CAD build for the part. Positions are in the model's coordinates, mm. A direction names the side the tool comes from. Give positions to 0.01 mm unless a question says otherwise; leave off trailing zeros. Loops run counter-clockwise (first coordinate to the right, second up) from the corner with the lowest first, then second, coordinate; pieces in that order, holes last. Notation, with made-up numbers: (-38, 18) - (21, 18) arc R23 cw to (21, 41) - close; hole circle Ø8 at (60, -14). An arc over 180 degrees is marked (long way). Return JSON: item names as keys, results as strings.
from build123d import *

# Parameters (mm, degrees)
BOX069_W          = 2
BOX069_H          = 2
BOX069_DEPTH      = 2
BOX070_W          = 2
BOX070_H          = 2
BOX070_DEPTH      = 2
CYLINDER040_R     = 0.75
CYLINDER040_DEPTH = 10
CYLINDER037_R     = 0.75
CYLINDER037_DEPTH = 10
BOX038_W          = 5
BOX038_H          = 11
BOX038_DEPTH      = 3.2
BOX003_W          = 4
BOX003_H          = 19
BOX003_DEPTH      = 5
FILLET_R          = 1
FILLET001_R       = 1
FILLET002_R       = 1
FILLET003_R       = 1


with BuildPart() as cubo069:
    # Box069 → Box069 (new body)
    with BuildSketch(Plane(origin=(-27, 67, 43), x_dir=(1, 0, 0), z_dir=(0, 0, 1))):
        with Locations((1, 1)):
            Rectangle(BOX069_W, BOX069_H)
    extrude(amount=BOX069_DEPTH)


with BuildPart() as cubo070:
    # Box070 → Box070 (new body)
    with BuildSketch(Plane(origin=(-27, 50, 43), x_dir=(1, 0, 0), z_dir=(0, 0, 1))):
        with Locations((1, 1)):
            Rectangle(BOX070_W, BOX070_H)
    extrude(amount=BOX070_DEPTH)


with BuildPart() as cilindro040:
    # Cylinder040 → Cylinder040 (new body)
    with BuildSketch(Plane(origin=(-26, 66, 42), x_dir=(1, 0, 0), z_dir=(0, 0, 1))):
        Circle(CYLINDER040_R)
    extrude(amount=CYLINDER040_DEPTH)


with BuildPart() as cilindro037:
    # Cylinder037 → Cylinder037 (new body)
    with BuildSketch(Plane(origin=(-26, 53, 42), x_dir=(1, 0, 0), z_dir=(0, 0, 1))):
        Circle(CYLINDER037_R)
    extrude(amount=CYLINDER037_DEPTH)


with BuildPart() as cubo038:
    # Box038 → Box038 (new body)
    with BuildSketch(Plane(origin=(-28.5, 54, 51), x_dir=(1, 0, 0), z_dir=(0, 0, 1))):
        with Locations((2.5, 5.5)):
            Rectangle(BOX038_W, BOX038_H)
    extrude(amount=BOX038_DEPTH)


with BuildPart() as fusion002044002:
    # Box003 → Box003 (new body)
    with BuildSketch(Plane(origin=(-2, 50, 45), x_dir=(1, 0, 0), z_dir=(0, 0, 1))):
        with Locations((2, 9.5)):
            Rectangle(BOX003_W, BOX003_H)
    extrude(amount=BOX003_DEPTH)

    # Fillet
    fillet_edges = [fusion002044002.edges().sort_by_distance(p)[0] for p in [
        (2, 59.5, 50),
    ]]
    fillet(fillet_edges, radius=FILLET_R)

    # Fillet001
    fillet001_edges = [fusion002044002.edges().sort_by_distance(p)[0] for p in [
        (-2, 59.5, 50),
    ]]
    fillet(fillet001_edges, radius=FILLET001_R)

    # Fillet002
    fillet002_edges = [fusion002044002.edges().sort_by_distance(p)[0] for p in [
        (0, 69, 50),
    ]]
    fillet(fillet002_edges, radius=FILLET002_R)

    # Fillet003
    fillet003_edges = [fusion002044002.edges().sort_by_distance(p)[0] for p in [
        (0, 50, 50),
    ]]
    fillet(fillet003_edges, radius=FILLET003_R)


with BuildPart() as fusion002044002_1:
    # Fillet003 placement: moved
    add(fusion002044002.part.moved(Location((-26, 0, 6))))

    # Cut055: cut Cubo038
    add(cubo038.part, mode=Mode.SUBTRACT)


with BuildPart() as fusion002044002_2:
    # Cut055 placement: moved
    add(fusion002044002_1.part.moved(Location((0, 0, -6))))

    # Cut057: cut Cilindro037
    add(cilindro037.part, mode=Mode.SUBTRACT)

    # Cut058: cut Cilindro040
    add(cilindro040.part, mode=Mode.SUBTRACT)

    # Fusion002044002: union Cubo069, Cubo070
    add(cubo069.part)
    add(cubo070.part)


solid = fusion002044002_2.part
1. Drop flat-ended pins along their axis: P1, Ø1.6, axis at y = 68, z = 43.5, coming from the +X side; P2, Ø1.4, axis at x = -26, y = 53, coming from the +Z side; P3, Ø2, axis at y = 68.5, z = 43.5, coming from the -X side. Give the stop position or say it passes through.
Values follow:
{"P1": "stops at x = -25", "P2": "passes through", "P3": "stops at x = -27"}
2. Cut at D-D, the plane z = 47.5. Write the cut outline in (x, y), plus the area to 3 significant figures.
Values follow:
{"outline": "(-28, 51) arc R1 ccw to (-27, 50) - (-25, 50) arc R1 ccw to (-24, 51) - (-24, 54) - (-28, 54) - close; (-28, 65) - (-24, 65) - (-24, 68) arc R1 ccw to (-25, 69) - (-27, 69) arc R1 ccw to (-28, 68) - close; hole circle Ø1.5 at (-26, 53); hole circle Ø1.5 at (-26, 66)", "area": "27.6 mm²"}
3. Drill centre lines: probe 1 along Y at (x, z) = (-26, 47.2); probe 2 along Y at (x, z) = (-26, 49.05); probe 3 along X at (y, z) = (66, 46.95). Where is each one in solid material? Low to high.
Values follow:
{"probe 1": "y = 50 to 52.25, 53.75 to 54, 65 to 65.25, 66.75 to 69", "probe 2": "y = 50 to 52.25, 53.75 to 65.25, 66.75 to 69", "probe 3": "x = -28 to -26.75, -25.25 to -24"}
4. Cut at C-C, the plane y = 66. Write the cut outline in (x, z).
Values follow:
{"outline": "(-28, 45) - (-26.75, 45) - (-26.75, 50) - (-27, 50) arc R1 ccw to (-28, 49) - close; (-25.25, 45) - (-24, 45) - (-24, 49) arc R1 ccw to (-25, 50) - (-25.25, 50) - close"}
5. Cut at A-A, the plane z = 44.5. Write the cut outline in (x, y), plus the area to 3 significant figures.
Values follow:
{"outline": "(-27, 50) - (-25, 50) - (-25, 52) - (-27, 52) - close; (-27, 67) - (-25, 67) - (-25, 69) - (-27, 69) - close", "area": "8.00 mm²"}
6. Pull direction Y, two halves, no side cores. Call faces 6 (the face through (-25.986, 50.301, 49.715)), 7 (the face through (-26, 65, 47)), 8 (the face through (-24, 59.4, 48.7)): +Y half, -Y half, draft (parallel to the pull), parting line (faces both ways), or undercut.
Values follow:
{"face 6": "-Y half", "face 7": "undercut", "face 8": "draft"}
7. Which spindle directions (+Z, -Z, +X, -X, +Y, -Y) get a long thin tool onto all of the face, cutting with end or side? Do faces 1 (the face through (-26, 50, 46)), 2 (the face through (-25, 68, 44)), 3 (the face through (-26, 52, 44)), 4 (the face through (-27, 68, 44)), 5 (the face through (-26, 51, 43)). Say none if no direction does.
Values follow:
{"face 1": "+Z, -Z, +X, -X, -Y", "face 2": "-Z, +X, +Y, -Y", "face 3": "-Z, +X, -X", "face 4": "-Z, -X, +Y, -Y", "face 5": "-Z, +X, -X, +Y, -Y"}
8. Cut at B-B, the plane x = -26. Write the cut outline in (y, z).
Values follow:
{"outline": "(50, 43) - (52, 43) - (52, 45) - (52.25, 45) - (52.25, 50) - (51, 50) arc R1 ccw to (50, 49) - close; (53.75, 45) - (54, 45) - (54, 48.2) - (65, 48.2) - (65, 45) - (65.25, 45) - (65.25, 50) - (53.75, 50) - close; (66.75, 45) - (67, 45) - (67, 43) - (69, 43) - (69, 49) arc R1 ccw to (68, 50) - (66.75, 50) - close"}
